Can you work these out from the model? Positions are in its coordinate system, mm. A direction names the side the tool comes from. Coordinates: 2 decimals unless noted, no trailing zeros. Order: outer loops, then holes, each group sorted by start corner. A loop starts at its lowest first (then second) coordinate and runs counter-clockwise, first axis right, second up. Notation, with made-up numbers: (71, 36.5) -> (107, 36.5) arc R29 cw to (107, 70.5) -> close; hole circle Ø11 at (-39, 64). An arc over 180 degrees is marked (long way). Return JSON: item names as keys, results as strings. Group by question number.
1) Thinking about a two-plate mould opening in Y: for faces 3 (the flat face through (3.464, 15, 5)), 4 (the flat face through (-3, 30, 0)), 5 (the cylindrical face through (-3.52, 5.79, -2.86)), which applies, +Y half, -Y half, draft (parallel to the pull), parting line (faces both ways), or undercut?
2) If we section it at B-B, the plane x = 1.25: Please give me the cut outline in (y, z), then the cut area to 3 significant figures.
3) If we section it at A-A, the plane y = 4.59: Please give me the cut outline in (x, z), then the cut area to 3 significant figures.
4) If we section it at C-C, the plane y = 18.25: Please give me the cut outline in (x, z).
5) For faces 1 (the flat face through (-3, 0, 0)), 2 (the flat face through (0, 15, 4.26)), which set-ups out of +Z, -Z, +X, -X, +Y, -Y let a thin tool reach every point of the face, with its end or its side?
6) If we section it at D-D, the plane z = -6.25: Please give me the cut outline in (x, y).
7) For pin 1 (3 mm diameter, centred on x = -0.5, y = 20.5, fed in from -Z); pin 2 (4.5 mm diameter, centred on y = 15, z = -4.5, fed in from +X), each with a flat end and sliding along its axis, tell me the tip position at first contact or that it passes through.
8) If I drill on probe 1 along X at (y, z) = (11.25, -5.75); probe 2 along Z at (x, y) = (0.5, 27.25); probe 3 along Z at (x, y) = (-3.25, 6), over which ranges is the centre line in solid material (lowest first)? Write a range as from..to.
from build123d import *

# Parameters (mm, degrees)
BOSS_EXTRUDE1_DEPTH = 30
SKETCH2_R           = 1.675
CUT_EXTRUDE1_DEPTH  = 30
SKETCH3_R           = 1.75
CUT_EXTRUDE2_DEPTH  = 30


with BuildPart() as part:
    # Sketch1 → Boss-Extrude1 (new body)
    with BuildSketch(Plane(origin=(0, 0, 0), x_dir=(1, 0, 0), z_dir=(0, 1, 0))):
        Polygon((-2.53610988, 10.739698715), (-2.53610988, -4.260301285), (3.46389012, -4.260301285), (3.46389012, -6.260301285), (-4.53610988, -6.260301285), (-4.53610988, 10.739698715), align=None)
    extrude(amount=BOSS_EXTRUDE1_DEPTH)

    # Sketch2 → Cut-Extrude1 (cut)
    with BuildSketch(Plane(origin=(0, 0, 4.260301285), x_dir=(-1, 0, 0), z_dir=(0, 0, -1))):
        with Locations((-0.63889012, 25.414)):
            Circle(SKETCH2_R)
        with Locations((-0.64389012, 4.59)):
            Circle(SKETCH2_R)
    extrude(amount=-CUT_EXTRUDE1_DEPTH, mode=Mode.SUBTRACT)

    # Sketch3 → Cut-Extrude2 (cut)
    with BuildSketch(Plane(origin=(-2.53610988, 0, 0), x_dir=(0, 0, -1), z_dir=(1, 0, 0))):
        with Locations((3.239698715, 22.5)):
            Circle(SKETCH3_R)
        with Locations((3.239698715, 7.5)):
            Circle(SKETCH3_R)
    extrude(amount=-CUT_EXTRUDE2_DEPTH, mode=Mode.SUBTRACT)


solid = part.part
Result sheet:
{
 "1": {"face 3": "draft", "face 4": "+Y half", "face 5": "undercut"},
 "2": {"outline": "(0, 4.26) -> (3.03, 4.26) -> (3.03, 6.26) -> (0, 6.26) -> close; (6.15, 4.26) -> (23.85, 4.26) -> (23.85, 6.26) -> (6.15, 6.26) -> close; (26.97, 4.26) -> (30, 4.26) -> (30, 6.26) -> (26.97, 6.26) -> close", "area": "47.5 mm2"},
 "3": {"outline": "(-4.54, -10.74) -> (-2.54, -10.74) -> (-2.54, 4.26) -> (-1.03, 4.26) -> (-1.03, 6.26) -> (-4.54, 6.26) -> close; (2.32, 4.26) -> (3.46, 4.26) -> (3.46, 6.26) -> (2.32, 6.26) -> close", "area": "39.3 mm2"},
 "4": {"outline": "(-4.54, -10.74) -> (-2.54, -10.74) -> (-2.54, 4.26) -> (3.46, 4.26) -> (3.46, 6.26) -> (-4.54, 6.26) -> close"},
 "5": {"face 1": "+Z, -Z, +X, -X, -Y", "face 2": "-Z, +X, +Y, -Y"},
 "6": {"outline": "(-4.54, 0) -> (-2.54, 0) -> (-2.54, 30) -> (-4.54, 30) -> close"},
 "7": {"pin 1": "stops at z = 4.26", "pin 2": "stops at x = -2.54"},
 "8": {"probe 1": "x = -4.54..-2.54", "probe 2": "z = 4.26..6.26", "probe 3": "z = -10.74..-4.14, -2.34..6.26"}
}
